```python
from build123d import *

# Parameters (mm, degrees)
F0_W     = 40
F0_H     = 9
F0_W_2   = 16.9967
F0_H_2   = 5
F1_DEPTH = 8
F2_R     = 1
F3_R     = 1


with BuildPart() as f1:
    # F0 (on Top) → F1 (new body)
    with BuildSketch(Plane.XY):
        Rectangle(F0_W, F0_H)
        with Locations((-9.50165, 0)):
            Rectangle(F0_W_2, F0_H_2, mode=Mode.SUBTRACT)
        with Locations((9.50165, 0)):
            Rectangle(F0_W_2, F0_H_2, mode=Mode.SUBTRACT)
    extrude(amount=F1_DEPTH)

    # F2
    f2_edges = [f1.edges().sort_by_distance(p)[0] for p in [
        (-20, -4.5, 4),
        (-20, 4.5, 4),
        (20, -4.5, 4),
        (20, 4.5, 4),
    ]]
    fillet(f2_edges, radius=F2_R)

    # F3
    f3_edges = [f1.edges().sort_by_distance(p)[0] for p in [
        (1.0033, -2.5, 4),
        (1.0033, 2.5, 4),
        (-1.0033, 2.5, 4),
        (-1.0033, -2.5, 4),
        (-18, -2.5, 4),
        (-18, 2.5, 4),
        (18, 2.5, 4),
        (18, -2.5, 4),
    ]]
    fillet(f3_edges, radius=F3_R)


solid = f1.part
```
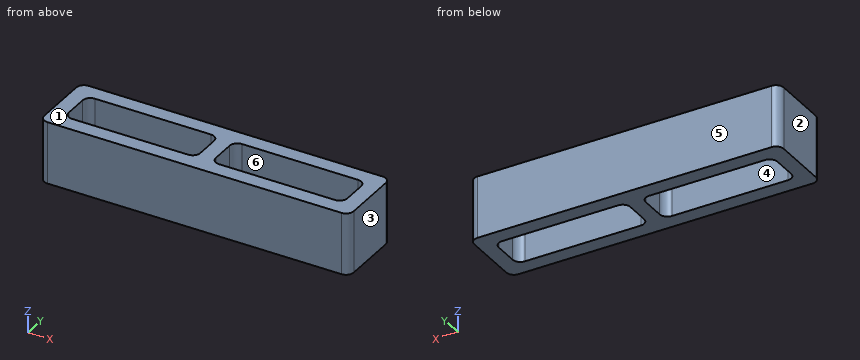
Verification items for the finished model (mm, model axes). Face numbers are marked on the shaded views. A direction names the side the tool comes from. Round coordinates to 2 decimals unless told otherwise and drop trailing zeros. Order: outer loops, then holes, each group sorted by start corner. A loop starts at its lowest first (then second) coordinate and runs counter-clockwise, first axis right, second up.
1) Cross-section at B-B, the plane z = 5.25. Record the cut outline in (x, y), plus the area to 3 significant figures.
Geometry says:
outline: (-20, -3.5) arc R1 ccw to (-19, -4.5) - (19, -4.5) arc R1 ccw to (20, -3.5) - (20, 3.5) arc R1 ccw to (19, 4.5) - (-19, 4.5) arc R1 ccw to (-20, 3.5) - close; hole (-18, -1.5) arc R1 ccw to (-17, -2.5) - (-2, -2.5) arc R1 ccw to (-1, -1.5) - (-1, 1.5) arc R1 ccw to (-2, 2.5) - (-17, 2.5) arc R1 ccw to (-18, 1.5) - close; hole (1, -1.5) arc R1 ccw to (2, -2.5) - (17, -2.5) arc R1 ccw to (18, -1.5) - (18, 1.5) arc R1 ccw to (17, 2.5) - (2, 2.5) arc R1 ccw to (1, 1.5) - close
area: 191 mm2
2) Tool access check on the marked faces 5 and 6. Record the directions out of +Z, -Z, +X, -X, +Y, -Y that give a thin tool (end or side, any length) a straight path to the whole face; none if there is none.
Geometry says:
face 5: +Z, -Z, +X, -X, +Y
face 6: +Z, -Z
3) Cross-section at A-A, the plane y = 0. Record the cut outline in (x, z), plus the area to 3 significant figures.
Geometry says:
outline: (-20, 0) - (-18, 0) - (-18, 8) - (-20, 8) - close; (-1, 0) - (1, 0) - (1, 8) - (-1, 8) - close; (18, 0) - (20, 0) - (20, 8) - (18, 8) - close
area: 48.1 mm2
4) Draft check along X on the marked faces 1, 2, 3 and 4. Enter one of: +X half, -X half, draft (parallel to the pull), parting line (faces both ways), or undercut.
Geometry says:
face 1: draft
face 2: -X half
face 3: +X half
face 4: undercut
5) Cross-section at D-D, the plane y = -2. Record the cut outline in (x, z), plus the area to 3 significant figures.
Geometry says:
outline: (-20, 0) - (-17.87, 0) - (-17.87, 8) - (-20, 8) - close; (-1.14, 0) - (1.14, 0) - (1.14, 8) - (-1.14, 8) - close; (17.87, 0) - (20, 0) - (20, 8) - (17.87, 8) - close
area: 52.3 mm2
6) Cross-section at C-C, the plane x = -7.5. Record the cut outline in (y, z), plus the area to 3 significant figures.
Geometry says:
outline: (-4.5, 0) - (-2.5, 0) - (-2.5, 8) - (-4.5, 8) - close; (2.5, 0) - (4.5, 0) - (4.5, 8) - (2.5, 8) - close
area: 32.0 mm2
7) Material ranges on line 1 (X direction, y = 1.25, z = 3); line 2 (Y direction, x = 3, z = 5); line 3 (X direction, y = -2.25, z = 5.75), recorded low to high.
Geometry says:
line 1: x = -20 to -18, -1 to 1, 18 to 20
line 2: y = -4.5 to -2.5, 2.5 to 4.5
line 3: x = -20 to -17.66, -1.34 to 1.34, 17.66 to 20
